Read the model definition and answer for the solid it produces. Units are mm, in the model's axes. Coordinates: 2 decimals unless noted, no trailing zeros. Order: outer loops, then holes, each group sorted by start corner. A loop starts at its lowest first (then second) coordinate and runs counter-clockwise, first axis right, second up.
```python
from build123d import *

# Parameters (mm, degrees)
SKETCH1_W                                = 70
SKETCH1_H                                = 80
BOSS_EXTRUDE1_DEPTH                      = 5
CUT_EXTRUDE1_START                       = -6
CUT_EXTRUDE1_DEPTH                       = 7
MIRROR1_START                            = -6
MIRROR1_AT_THE_SECOND_PLANE_COPY_1_DEPTH = 7
SKETCH4_R                                = 1.5875
CUT_EXTRUDE2_DEPTH                       = 6


with BuildPart() as part:
    # Sketch1 → Boss-Extrude1 (new body)
    with BuildSketch(Plane(origin=(0, 0, 0), x_dir=(0, 0, -1), z_dir=(1, 0, 0))):
        Rectangle(SKETCH1_W, SKETCH1_H)
    extrude(amount=BOSS_EXTRUDE1_DEPTH)

    # Sketch3 → Cut-Extrude1 (cut)
    with BuildSketch(Plane(origin=(5, 0, 0), x_dir=(0, 0, -1), z_dir=(1, 0, 0)).offset(CUT_EXTRUDE1_START)):
        Polygon((-35, 20), (-30, 20), (-30, 35), (-15, 35), (-15, 40), (-35, 40), align=None)
    cut_extrude1 = extrude(amount=CUT_EXTRUDE1_DEPTH, mode=Mode.SUBTRACT)

    # Mirror1: Cut-Extrude1 across plane
    add(cut_extrude1.mirror(Plane.XY), mode=Mode.SUBTRACT)

    # Mirror1 at the second plane: Cut-Extrude1 across plane
    add(cut_extrude1.mirror(Plane.ZX), mode=Mode.SUBTRACT)

    # Mirror1 at the second plane copy 1 sketc → Mirror1 at the second plane copy 1 (cut)
    with BuildSketch(Plane(origin=(5, 0, 0), x_dir=(0, 0, 1), z_dir=(1, 0, 0)).offset(MIRROR1_START)):
        Polygon((-35, 20), (-30, 20), (-30, 35), (-15, 35), (-15, 40), (-35, 40), align=None)
    extrude(amount=MIRROR1_AT_THE_SECOND_PLANE_COPY_1_DEPTH, mode=Mode.SUBTRACT)

    # Sketch4 → Cut-Extrude2 (cut, through all)
    with BuildSketch(Plane(origin=(5, 0, 0), x_dir=(0, 0, -1), z_dir=(1, 0, 0))):
        with Locations((-30, 20)):
            Circle(SKETCH4_R)
        with Locations((-15, 35)):
            Circle(SKETCH4_R)
        with Locations((15, 35)):
            Circle(SKETCH4_R)
        with Locations((30, 20)):
            Circle(SKETCH4_R)
        with Locations((30, -20)):
            Circle(SKETCH4_R)
        with Locations((15, -35)):
            Circle(SKETCH4_R)
        with Locations((-15, -35)):
            Circle(SKETCH4_R)
        with Locations((-30, -20)):
            Circle(SKETCH4_R)
    extrude(amount=-CUT_EXTRUDE2_DEPTH, mode=Mode.SUBTRACT)


solid = part.part
```
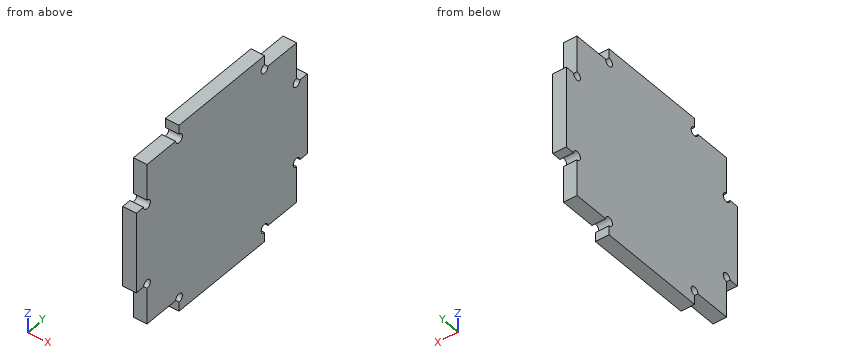
1) A cutting plane is placed at C-C, the plane z = 17.5. Determine the outline of the cut face in (x, y), and give its area (3 significant figures).
A:
outline: (0, -35) - (5, -35) - (5, 35) - (0, 35) - close
area: 350 mm2
2) Straight lines are drawn through the part: line 1 (Z direction, x = 2.4, y = 34.5); line 2 (Z direction, x = 2, y = 23); line 3 (Y direction, x = 3.95, z = 28). For each, find the intervals that lie inside material, in ascending order.
A:
line 1: z = -30 to -16.51, -13.49 to 13.49, 16.51 to 30
line 2: z = -30 to 30
line 3: y = -35 to 35
3) Flat-ended cylindrical pins translate along their axes: pin 1 Ø1.5 at (x, y) = (1.5, 30) entering from -Z; pin 2 Ø1.5 at (x, z) = (2.5, -20.5) entering from -Y; pin 3 Ø2.5 at (x, z) = (3, 22) entering from +Y. Find the tip coordinate at first contact, or state that the pin passes through.
A:
pin 1: stops at z = -30
pin 2: stops at y = -35
pin 3: stops at y = 35
4) A cutting plane is placed at B-B, the plane y = -28.5. Determine the outline of the cut face in (x, z), and give its area (3 significant figures).
A:
outline: (0, -30) - (5, -30) - (5, 30) - (0, 30) - close
area: 300 mm2
5) A cutting plane is placed at A-A, the plane x = 2.4. Determine the outline of the cut face in (y, z) (1 decimal), and give its area (3 significant figures).
A:
outline: (-40, -15) - (-36.6, -15) arc R1.6 cw (long way) to (-35, -16.6) - (-35, -30) - (-21.6, -30) arc R1.6 cw (long way) to (-20, -31.6) - (-20, -35) - (20, -35) - (20, -31.6) arc R1.6 cw (long way) to (21.6, -30) - (35, -30) - (35, -16.6) arc R1.6 cw (long way) to (36.6, -15) - (40, -15) - (40, 15) - (36.6, 15) arc R1.6 cw (long way) to (35, 16.6) - (35, 30) - (21.6, 30) arc R1.6 cw (long way) to (20, 31.6) - (20, 35) - (-20, 35) - (-20, 31.6) arc R1.6 cw (long way) to (-21.6, 30) - (-35, 30) - (-35, 16.6) arc R1.6 cw (long way) to (-36.6, 15) - (-40, 15) - close
area: 4,850 mm2
